from build123d import *

# Parameters (mm, degrees)
F0_R      = 20.2439763863
F1_DEPTH  = 10.16
F2_R      = 12.3390116376
F3_DEPTH  = 8.89
F5_DEPTH  = 0.254
F6_DEPTH  = 0.254
F7_DEPTH  = 2.286
F8_DEPTH  = 2.286
F10_DEPTH = 25.4
F11_DEPTH = 50.8
F12_DEPTH = 1.27
F13_DEPTH = 1.27
F14_DEPTH = 25.4


with BuildPart() as f1:
    # F0 (on Top) → F1 (new body)
    with BuildSketch(Plane.XY):
        Circle(F0_R)
    extrude(amount=F1_DEPTH)

    # F2 (on face) → F3 (join)
    with BuildSketch(Plane.XY.offset(10.16)):
        Circle(F2_R)
    extrude(amount=F3_DEPTH)

    # F4 (on Front) → F5 (join)
    with BuildSketch(Plane.XZ):
        with BuildLine():
            add(Edge.make_bspline(
                [(-12.1147008613, 18.9316812903), (-12.5825885387, 39.643614737), (-14.1043760911, 180.4872847527), (-20.1423116849, 215.1594423433), (-16.5980636671, 214.2285434237), (-12.8136342596, 217.1071550637), (-13.8994905387, 225.3991797656), (-17.690195851, 229.7737918888), (-21.3235962144, 228.5443351063), (-21.72468447, 231.1706865689), (-23.0745608098, 250.4649690024), (-22.9518555989, 256.8313726894), (-25.9612755155, 279.5145026457), (-19.7421258922, 272.3476049684), (-8.8885956952, 268.998501799), (6.6271937698, 261.4946225406), (12.2027765589, 256.1934321206), (17.5689411606, 248.9539384021), (19.5820695948, 242.6412768865), (21.7285943019, 235.2163703421), (21.0795757322, 226.6989574981), (17.1180518063, 124.7114584437), (15.2094878956, 77.70771609), (11.6083548837, 18.1667354361), (12.5199184163, 13.1739974773), (7.8980496645, 11.3722942506), (0.3726356815, 13.3748423837), (-11.8699226938, 12.3427906017), (-12.0266797417, 15.035259866), (-12.1147008613, 18.9316812903)],
                knots=[0, 0, 0, 0, 0.1257254435, 0.1801466998, 0.1919036578, 0.2112403794, 0.2389108592, 0.261334308, 0.2775826335, 0.2907551098, 0.3325149493, 0.3636705446, 0.4039783899, 0.4240659342, 0.4586729556, 0.4992031799, 0.5266476396, 0.5552636706, 0.5809163826, 0.6063516787, 0.6344015668, 0.7303572224, 0.8074506533, 0.8789177389, 0.897509656, 0.9162026247, 0.9446563322, 0.976347968, 1, 1, 1, 1], degree=3))
        make_face()
    extrude(amount=F5_DEPTH)

    # F6 (add): a face of the model
    f6_faces = [f1.faces().sort_by_distance(p)[0] for p in [
        (0.2349858377, 0, 153.5959306446),
    ]]
    extrude(f6_faces, amount=F6_DEPTH)

    # F7 (add): a face of the model
    f7_faces = [f1.faces().sort_by_distance(p)[0] for p in [
        (0.2349858377, 0.254, 153.5959306446),
    ]]
    extrude(f7_faces, amount=F7_DEPTH)

    # F8 (add): a face of the model
    f8_faces = [f1.faces().sort_by_distance(p)[0] for p in [
        (0.2349858377, -0.254, 153.5959306446),
    ]]
    extrude(f8_faces, amount=F8_DEPTH)

    # F9 (on Front) → F10 (join)
    with BuildSketch(Plane.XZ):
        Polygon((-28.4392070025, 277.075022459), (5.8726719581, 261.9545459747), (-7.6194559224, 282.5416624546), align=None)
    extrude(amount=F10_DEPTH)

    # F11 (cut): a face of the model
    f11_faces = [f1.faces().sort_by_distance(p)[0] for p in [
        (-10.061996989, -25.4, 273.8570769628),
    ]]
    extrude(f11_faces, amount=-F11_DEPTH, mode=Mode.SUBTRACT)

    # F12 (cut): a face of the model
    f12_faces = [f1.faces().sort_by_distance(p)[0] for p in [
        (0.248434517, -2.54, 153.5481680876),
    ]]
    extrude(f12_faces, amount=-F12_DEPTH, mode=Mode.SUBTRACT)

    # F13 (cut): a face of the model
    f13_faces = [f1.faces().sort_by_distance(p)[0] for p in [
        (0.248434517, 2.54, 153.5481680876),
    ]]
    extrude(f13_faces, amount=-F13_DEPTH, mode=Mode.SUBTRACT)

    # F14 (cut): a face of the model
    f14_faces = [f1.faces().sort_by_distance(p)[0] for p in [
        (0.248434517, -1.27, 153.5481680876),
    ]]
    extrude(f14_faces, amount=-F14_DEPTH, mode=Mode.SUBTRACT)


solid = f1.part
Model file for the job. Use its own axes, mm. A direction names the side the tool comes from. Coordinates: 2 decimals unless noted, no trailing zeros. Write each loop counter-clockwise with the first axis right and the second up, starting at its lowest first coordinate (ties: lowest second). Pieces come first, ordered by that corner, then holes. Notation, with made-up numbers: (-24, -1.5) - (3, -1.5) arc R23 cw to (3, 13.5) - close; hole circle Ø7 at (39.25, 79). An arc over 180 degrees is marked (long way). Write each question's results on one line, items separated by ' | '. Start each with the question number.
1) Cut at D-D (y = 13). Write the cut outline in (x, z), then the cut area to 3 significant figures.
2) Cut at A-A (x = 0). Write the cut outline in (y, z).
3) Flat gauge pins, fed straight in: P1, Ø6, axis at y = -12.5, z = 15.5, coming from the -X side; P2, Ø2, axis at y = -1.5, z = 11, coming from the +X side; P3, Ø2, axis at x = -8, z = 14.5, coming from the +Y side; P4, Ø1, axis at y = -13.5, z = 11.5, coming from the -X side. Where does each tip first touch, or does it go through?
4) Cut at C-C (z = 15.75). Write the cut outline in (x, y), then the cut area to 3 significant figures.
5) 3-axis set-ups, long thin cutter, end or side, ignore diameter. For faces 1 (the face through (19.31, 6.08, 5.01)), 2 (the face through (-9, -9, 10.16)): which of +Z, -Z, +X, -X, +Y, -Y reach the whole face in a straight line?
6) Probe line 1 along Z through (x, y) = (-6, -18); line 2 along X through (y, z) = (-4.5, 13); line 3 along Y through (x, z) = (-10.5, 16). List the from-to ranges inside material, lowest first. Write a range as from..to.
Returned:
1) outline: (-15.52, 0) - (15.52, 0) - (15.52, 10.16) - (-15.52, 10.16) - close | area: 315 mm^2
2) outline: (-20.24, 0) - (20.24, 0) - (20.24, 10.16) - (12.34, 10.16) - (12.34, 19.05) - (-12.34, 19.05) - (-12.34, 10.16) - (-20.24, 10.16) - close
3) P1: x = -7.87 | P2: x = 20.22 | P3: y = 10.16 | P4: through
4) outline: circle Ø24.68 at (0, 0) | area: 478 mm^2
5) face 1: +Z, -Z | face 2: +Z
6) line 1: 0..10.16 | line 2: -11.49..11.49 | line 3: -6.48..6.48
